Work out the finished part from the listing and answer in its coordinate system (mm). Face numbers are marked on the shaded views. Round coordinates to 2 decimals unless told otherwise and drop trailing zeros. Write each loop counter-clockwise with the first axis right and the second up, starting at its lowest first coordinate (ties: lowest second). Pieces come first, ordered by that corner, then holes.
1. Find section C-C (x = -1). Write down the section's boundary in (y, z).
2. Find section A-A (y = 4). Write down the section's boundary in (x, z).
3. Determine the mould class of the marked faces 1, 2 and 3 for opening direction Z: pulls with the +Z half, pulls with the -Z half, needs draft (parallel to the pull), parting line crosses it, or undercut.
4. Find section D-D (z = 3). Write down the section's boundary in (x, y), and give its area (3 significant figures).
5. Straight lines are drawn through the part: probe 1 along Y at (x, z) = (7.75, -3); probe 2 along Z at (x, y) = (0, 2.9). For each, find the intervals that lie inside material, in ascending order.
6. Find section B-B (z = 0). Write down the section's boundary in (x, y), and give its area (3 significant figures).
7. A flat-ended cylindrical pin translates along its axis: pin 1 Ø1 at (y, z) = (3.5, 6.5) entering from -X. Find the tip coordinate at first contact, or state that the pin passes through.
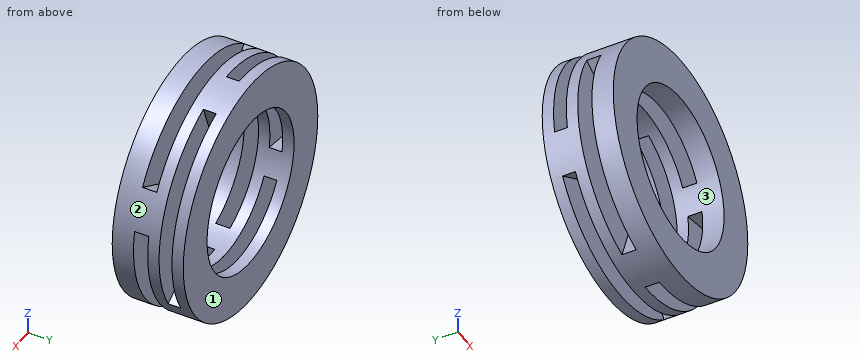
```python
from build123d import *

# Parameters (mm, degrees)
ESBO_O9_W             = 3
ESBO_O9_H             = 5
CORTE_EXTRUS_O1_DEPTH = 1
PADR_OCIRCULAR2_COUNT = 3
CORTE_EXTRUS_O3_START = 0.9
CORTE_EXTRUS_O3_DEPTH = 0.9
PADR_OCIRCULAR4_COUNT = 3


with BuildPart() as part:
    # Esboço9 → Revolução1 (revolve)
    with BuildSketch(Plane.XY, mode=Mode.PRIVATE) as revolu_o1_sk:
        with Locations((7, 2.5)):
            Rectangle(ESBO_O9_W, ESBO_O9_H)
    revolve(revolu_o1_sk.sketch.rotate(Axis((0, -112.760074913, 0), (0, 1, 0)), 180), axis=Axis((0, -112.760074913, 0), (0, 1, 0)))

    # Esboço12 → Corte-extrusão1 (cut)
    with BuildSketch(Plane(origin=(0, 1.5, 0), x_dir=(1, 0, 0), z_dir=(0, 1, 0))):
        with BuildLine():
            Line((0, 8.5), (0, 5.5))
            ThreePointArc((0, 5.5), (4.213244437, 3.535331853), (5.416442642, -0.955064977))
            Line((5.416442642, -0.955064977), (8.370865901, -1.47600951))
            ThreePointArc((8.370865901, -1.47600951), (6.511377767, 5.463694682), (0, 8.5))
        make_face()
    corte_extrus_o1 = extrude(amount=CORTE_EXTRUS_O1_DEPTH, mode=Mode.SUBTRACT)

    # PadrãoCircular2: Corte-extrusão1 ×3 about axis
    padr_ocircular2_axis = Axis((0, 0, 0), (0, 1, 0))
    for i in range(1, PADR_OCIRCULAR2_COUNT):
        add(corte_extrus_o1.rotate(padr_ocircular2_axis, i * 360 / PADR_OCIRCULAR2_COUNT), mode=Mode.SUBTRACT)

    # Esboço13 → Corte-extrusão3 (cut)
    with BuildSketch(Plane(origin=(0, 3.3, 0), x_dir=(1, 0, 0), z_dir=(0, 1, 0)).offset(CORTE_EXTRUS_O3_START)):
        with BuildLine():
            Line((0, 0), (7.361215932, 4.25))
            ThreePointArc((7.361215932, 4.25), (7.987387277, -2.907171218), (2.907171218, -7.987387277))
            Line((2.907171218, -7.987387277), (0, 0))
        make_face()
    corte_extrus_o3 = extrude(amount=-CORTE_EXTRUS_O3_DEPTH, mode=Mode.SUBTRACT)

    # PadrãoCircular4: Corte-extrusão3 ×3 about axis
    padr_ocircular4_axis = Axis((0, 0, 0), (0, 1, 0))
    for i in range(1, PADR_OCIRCULAR4_COUNT):
        add(corte_extrus_o3.rotate(padr_ocircular4_axis, i * 360 / PADR_OCIRCULAR4_COUNT), mode=Mode.SUBTRACT)


solid = part.part
```
Worked answers:
1. outline: (0, -8.44) - (3.3, -8.44) - (3.3, -5.41) - (0, -5.41) - close; (0, 5.41) - (1.5, 5.41) - (1.5, 8.44) - (0, 8.44) - close; (2.5, 5.41) - (3.3, 5.41) - (3.3, 8.44) - (2.5, 8.44) - close; (4.2, -8.44) - (5, -8.44) - (5, -5.41) - (4.2, -5.41) - close; (4.2, 5.41) - (5, 5.41) - (5, 8.44) - (4.2, 8.44) - close
2. outline: (-8.37, -1.48) arc R8.5 ccw to (-7.36, -4.25) - (-4.76, -2.75) arc R5.5 cw to (-5.42, -0.96) - close; (0, 5.5) arc R5.5 cw to (1.88, 5.17) - (2.91, 7.99) arc R8.5 ccw to (0, 8.5) - close; (3.54, -4.21) - (5.46, -6.51) arc R8.5 ccw to (7.36, -4.25) - (4.76, -2.75) arc R5.5 cw to start
3. face 1: needs draft
3. face 2: parting line crosses it
3. face 3: undercut
4. outline: (-7.95, 0) - (-4.61, 0) - (-4.61, 3.3) - (-7.95, 3.3) - (-7.95, 2.5) - (-5.2, 2.5) - (-5.2, 1.5) - (-7.95, 1.5) - close; (-7.95, 4.2) - (-4.61, 4.2) - (-4.61, 5) - (-7.95, 5) - close; (4.61, 0) - (7.95, 0) - (7.95, 3.3) - (4.61, 3.3) - (4.61, 2.5) - (5.2, 2.5) - (5.2, 1.5) - (4.61, 1.5) - close; (4.61, 4.2) - (7.95, 4.2) - (7.95, 5) - (4.61, 5) - close
4. area: 24.1 mm2
5. probe 1: y = 0 to 1.5, 2.5 to 3.3, 4.2 to 5
5. probe 2: z = -8.5 to -5.5, 5.5 to 8.5
6. outline: (-8.5, 0) - (-5.5, 0) - (-5.5, 1.5) - (-8.5, 1.5) - close; (-8.5, 2.5) - (-5.5, 2.5) - (-5.5, 3.3) - (-8.5, 3.3) - close; (-8.5, 4.2) - (-5.5, 4.2) - (-5.5, 5) - (-8.5, 5) - close; (5.5, 0) - (8.5, 0) - (8.5, 1.5) - (5.5, 1.5) - close; (5.5, 2.5) - (8.5, 2.5) - (8.5, 3.3) - (5.5, 3.3) - close; (5.5, 4.2) - (8.5, 4.2) - (8.5, 5) - (5.5, 5) - close
6. area: 18.6 mm2
7. pin 1: stops at x = -5.98
